Read the model definition and answer for the solid it produces. Units are mm, in the model's axes. Round coordinates to 2 decimals unless told otherwise and drop trailing zeros. Order: outer loops, then holes, each group sorted by start corner. A loop starts at its lowest first (then second) coordinate and runs counter-clockwise, first axis right, second up. Notation, with made-up numbers: M 76,40 L 128,40 A15 cw 128,57 Z; hole C -34,60 d11. An arc over 180 degrees is marked long. Use one line per item in the form item = value. Start each with the question number.
from build123d import *

# Parameters (mm, degrees)
SKETCH_1_W          = 10
SKETCH_1_H          = 10
SKETCH_1_W_2        = 8
SKETCH_1_H_2        = 8
EXTRUDE_1_DEPTH     = 183
SKETCH_2_R          = 1.75
SKETCH_2_R_2        = 1.5
CUT_EXTRUDE_1_DEPTH = 11
SKETCH_4_R          = 1.5
CUT_EXTRUDE_2_DEPTH = 5


with BuildPart() as part:
    # 草图1 → 拉伸-薄壁1 (new body)
    with BuildSketch(Plane.XY):
        Rectangle(SKETCH_1_W, SKETCH_1_H)
        Rectangle(SKETCH_1_W_2, SKETCH_1_H_2, mode=Mode.SUBTRACT)
    extrude(amount=EXTRUDE_1_DEPTH)

    # 草图2 → 切除-拉伸1 (cut, through all)
    with BuildSketch(Plane(origin=(0, 5, 0), x_dir=(1, 0, 0), z_dir=(0, 1, 0))):
        Polygon((5, -183), (5, -178), (0, -183), align=None)
        with Locations((0, -178.0520382)):
            Circle(SKETCH_2_R)
        with Locations((0, -168)):
            Circle(SKETCH_2_R_2)
        with Locations((0, -128)):
            Circle(SKETCH_2_R_2)
        with Locations((0, -117.9479618)):
            Circle(SKETCH_2_R)
        with Locations((0, -80.5)):
            Circle(SKETCH_2_R_2)
        with Locations((0, -65.5)):
            Circle(SKETCH_2_R_2)
        with Locations((0, -53)):
            Circle(SKETCH_2_R_2)
    extrude(amount=-CUT_EXTRUDE_1_DEPTH, mode=Mode.SUBTRACT)

    # 草图4 → 切除-拉伸2 (cut)
    with BuildSketch(Plane.ZY.offset(5)):
        with Locations((177, 0)):
            Circle(SKETCH_4_R)
    extrude(amount=-CUT_EXTRUDE_2_DEPTH, mode=Mode.SUBTRACT)


solid = part.part
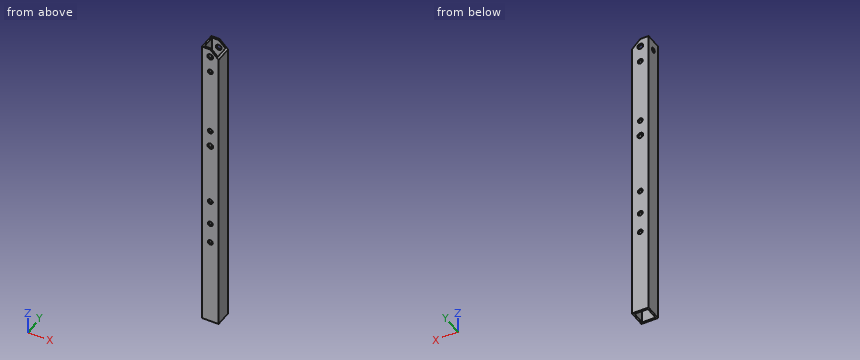
Item 1: Section A-A (z = 128) is taken. Write down the section's boundary in (x, y).
Item 2: Given P1, Ø2.5, axis at y = 0, z = 177, coming from the -X side, flat-ended and moving along its own axis, determine where the tip first touches the part or whether it passes through.
Item 3: Find the intervals of material crossed by L1, parallel to Y at x = -4.5, z = 177; L2, parallel to Y at x = 0.5, z = 11, in increasing order. Write a range as [from, to].
The answers:
q1.outline = M -5,-5 L -1.5,-5 L -1.5,-4 L -4,-4 L -4,4 L -1.5,4 L -1.5,5 L -5,5 Z; M 1.5,-5 L 5,-5 L 5,5 L 1.5,5 L 1.5,4 L 4,4 L 4,-4 L 1.5,-4 Z
q2.P1 = 4
q3.L1 = [-5, -1.5], [1.5, 5]
q3.L2 = [-5, -4], [4, 5]
